```python
from build123d import *

# Parameters (mm, degrees)
SKETCH1_R                          = 15.875
BOSS_EXTRUDE1_DEPTH                = 698.5
SKETCH2_R                          = 6.35
BOSS_EXTRUDE2_DEPTH                = 12.7
BOSS_EXTRUDE3_START                = 12.7
SKETCH3_R                          = 6.35
BOSS_EXTRUDE3_DEPTH                = 12.7
CBORE_FOR_M6_HEX_HEAD1_D           = 6.6
CBORE_FOR_M6_HEX_HEAD1_DEPTH       = 304.8
CBORE_FOR_M6_HEX_HEAD1_CBORE_D     = 14.547
CBORE_FOR_M6_HEX_HEAD1_CBORE_DEPTH = 4
CBORE_FOR_M6_HEX_HEAD1_TIP         = 1.982840043
CBORE_FOR_M6_HEX_HEAD4_D           = 6.6
CBORE_FOR_M6_HEX_HEAD4_DEPTH       = 304.8
CBORE_FOR_M6_HEX_HEAD4_CBORE_D     = 14.547
CBORE_FOR_M6_HEX_HEAD4_CBORE_DEPTH = 4
CBORE_FOR_M6_HEX_HEAD4_TIP         = 1.982840043


with BuildPart() as part:
    # Sketch1 → Boss-Extrude1 (new body)
    with BuildSketch(Plane.XY):
        Circle(SKETCH1_R)
    extrude(amount=BOSS_EXTRUDE1_DEPTH)

    # Sketch2 → Boss-Extrude2 (add)
    with BuildSketch(Plane.XY.offset(698.5)):
        Circle(SKETCH2_R)
    extrude(amount=BOSS_EXTRUDE2_DEPTH)

    # Sketch3 → Boss-Extrude3 (add)
    with BuildSketch(Plane(origin=(0, 0, 0), x_dir=(-1, 0, 0), z_dir=(0, 0, -1)).offset(BOSS_EXTRUDE3_START)):
        with Locations(Location((0, 0, 0), (0, 0, 180))):
            Circle(SKETCH3_R)
    extrude(amount=-BOSS_EXTRUDE3_DEPTH)

    # CBORE for M6 Hex Head1
    with Locations(Plane.XY.offset(711.2)):
        with Locations((0, 0)):
            CounterBoreHole(CBORE_FOR_M6_HEX_HEAD1_D / 2, CBORE_FOR_M6_HEX_HEAD1_CBORE_D / 2, CBORE_FOR_M6_HEX_HEAD1_CBORE_DEPTH, depth=CBORE_FOR_M6_HEX_HEAD1_DEPTH)
            with Locations((0, 0, -(CBORE_FOR_M6_HEX_HEAD1_DEPTH + CBORE_FOR_M6_HEX_HEAD1_TIP / 2))):  # 118° drill point
                Cone(0, CBORE_FOR_M6_HEX_HEAD1_D / 2, CBORE_FOR_M6_HEX_HEAD1_TIP, mode=Mode.SUBTRACT)

    # CBORE for M6 Hex Head4
    with Locations(Plane(origin=(0, 0, -12.7), x_dir=(-1, 0, 0), z_dir=(0, 0, -1))):
        with Locations((0, 0)):
            CounterBoreHole(CBORE_FOR_M6_HEX_HEAD4_D / 2, CBORE_FOR_M6_HEX_HEAD4_CBORE_D / 2, CBORE_FOR_M6_HEX_HEAD4_CBORE_DEPTH, depth=CBORE_FOR_M6_HEX_HEAD4_DEPTH)
            with Locations((0, 0, -(CBORE_FOR_M6_HEX_HEAD4_DEPTH + CBORE_FOR_M6_HEX_HEAD4_TIP / 2))):  # 118° drill point
                Cone(0, CBORE_FOR_M6_HEX_HEAD4_D / 2, CBORE_FOR_M6_HEX_HEAD4_TIP, mode=Mode.SUBTRACT)


solid = part.part
```
The model under review builds one solid part; all positions refer to its coordinate system, in mm. A direction names the side the tool comes from. Round coordinates to 2 decimals unless told otherwise and drop trailing zeros. Order: outer loops, then holes, each group sorted by start corner. A loop starts at its lowest first (then second) coordinate and runs counter-clockwise, first axis right, second up. Notation, with made-up numbers: M 25,-11 L 82,-11 A32 cw 82,27 Z; hole C 61,53.25 d2. An arc over 180 degrees is marked long. Use a Markdown table: item, result.
1) Consider section A-A (z = 537). Write out the cut boundary in (x, y) (3 decimals), then the cut area to 3 significant figures.
Report:
| item | result |
|---|---|
| outline | C 0,0 d31.75; hole C 0,0 d6.6 |
| area | 758 mm^2 |
2) Tool access review of faces 1 (the face through (7, 0, 698.5)), 2 (the face through (7, 0, 0)), 3 (the face through (-3, -3, -8.7)): name each direction out of +Z, -Z, +X, -X, +Y, -Y from which nothing blocks a thin tool from reaching the whole face with its end or side.
Report:
| item | result |
|---|---|
| face 1 | +Z |
| face 2 | -Z |
| face 3 | -Z, +X, -X, +Y, -Y |
3) Wall thickness on line 1 along X through (y, z) = (-0.5, 472.5); line 2 along Y through (x, z) = (0, 157) (3 decimals); line 3 along X through (y, z) = (1, 365): over which ranges is each line inside the solid? List them lowest first. Write a range as [from, to].
Report:
| item | result |
|---|---|
| line 1 | [-15.87, -3.26], [3.26, 15.87] |
| line 2 | [-15.875, -3.3], [3.3, 15.875] |
| line 3 | [-15.84, 15.84] |
4) Insertion check: pin 1 (1.5 mm diameter, centred on y = -7.5, z = 488.5, fed in from +X); pin 2 (1.5 mm diameter, centred on y = 5, z = 113, fed in from -X); pin 3 (1 mm diameter, centred on x = -2, y = 11.5, fed in from -Z). Each pin has a flat end and moves straight along its axis. Give the tip position at first contact, or say it passes through.
Report:
| item | result |
|---|---|
| pin 1 | x = 14.37 |
| pin 2 | x = -15.3 |
| pin 3 | z = 0 |
